from build123d import *

# Parameters (mm, degrees)
BOSS_EXTRUDE1_DEPTH = 31.75
SKETCH2_R           = 1.5
CUT_EXTRUDE1_DEPTH  = 183.851374072
FILLET1_R           = 10


with BuildPart() as part:
    # Sketch1 → Boss-Extrude1 (new body)
    with BuildSketch(Plane(origin=(0, 0, 0), x_dir=(1, 0, 0), z_dir=(0, 1, 0))):
        Polygon((0, 0), (-85, 0), (-85, 158.75), (0, 158.75), (0, 155.575), (-81.825, 155.575), (-81.825, 3.175), (0, 3.175), align=None)
    extrude(amount=BOSS_EXTRUDE1_DEPTH)

    # Sketch2 → Cut-Extrude1 (cut, through all)
    with BuildSketch(Plane.XY):
        with Locations((-7.5, 11.1125)):
            Circle(SKETCH2_R)
        with Locations((-7.5, 20.6375)):
            Circle(SKETCH2_R)
    extrude(amount=-CUT_EXTRUDE1_DEPTH, mode=Mode.SUBTRACT)

    # Fillet1
    fillet1_edges = [part.edges().sort_by_distance(p)[0] for p in [
        (-85, 15.875, 0),
        (-85, 15.875, -158.75),
        (-81.825, 15.875, -155.575),
        (-81.825, 15.875, -3.175),
    ]]
    fillet(fillet1_edges, radius=FILLET1_R)


solid = part.part
Input: part model. Units: mm. Frame: model coordinates. A direction names the side the tool comes from. Give positions to 0.01 mm unless a question says otherwise; leave off trailing zeros. Loops run counter-clockwise (first coordinate to the right, second up) from the corner with the lowest first, then second, coordinate; pieces in that order, holes last. Notation, with made-up numbers: (-2, 72) - (7, 72) arc R27 ccw to (7, 96) - close; hole circle Ø11 at (86, 21). An arc over 180 degrees is marked (long way). Use CSV: the item, a comma, the result in double quotes. Start each with the question number.
Item 1: Section D-D on z = -81. Return loops of the section in (x, y) (3 decimals).
Item 2: Line query: line 1 (Y direction, x = -7.5, z = -157.65); line 2 (Z direction, x = -37.5, y = 3.5) (3 decimals); line 3 (X direction, y = 20, z = -125) (3 decimals). Output: solid intervals per line, ascending.
Item 3: Contact query for flat-ended pins moving along their axis: P1, Ø1.5, axis at y = 3.5, z = -97, coming from the +X side (3 decimals); P2, Ø4, axis at x = -7.5, y = 11.11, coming from the -Z side. Output: stop coordinate, or through.
Item 4: Reachability of faces 1 (the flat face through (-36, 16, -3.175)), 2 (the cylindrical face through (-7.695, 22.125, -1.565)) from +Z, -Z, +X, -X, +Y, -Y: full face, straight path, thin tool, end or side. Return the list, or none.
Item 5: Mould query, pull axis Y, two halves, no side actions, for faces 3 (the flat face through (-37, 16, 0)), 4 (the cylindrical face through (-7.695, 22.125, -157.14)), 5 (the flat face through (-83, 31.75, -115)). Classes: pulls with the +Y half, pulls with the -Y half, needs draft (parallel to the pull), parting line crosses it, or undercut.
Item 6: Section B-B on x = -7.5. State how many separate pieces and enclosed holes the cut face has, then the cut area to 3 significant figures.
Item 7: Section A-A on x = -20. Return loops of the section in (y, z) (3 decimals), then the cut area to 3 significant figures.
Item 8: Section C-C on y = 6. Return loops of the section in (x, z) (3 decimals), then the cut area to 3 significant figures.
Ans:
1,outline,"(-85, 0) - (-81.825, 0) - (-81.825, 31.75) - (-85, 31.75) - close"
2,line 1,"y = 0 to 9.61, 12.61 to 19.14, 22.14 to 31.75"
2,line 2,"z = -158.75 to -155.575, -3.175 to 0"
2,line 3,"x = -85 to -81.825"
3,P1,"stops at x = -81.825"
3,P2,"stops at z = -158.75"
4,face 1,"+X, +Y, -Y"
4,face 2,"+Z, -Z"
5,face 3,"needs draft"
5,face 4,"undercut"
5,face 5,"pulls with the +Y half"
6,separate pieces,"6"
6,enclosed holes,"0"
6,area,"164 mm2"
7,outline,"(0, -158.75) - (31.75, -158.75) - (31.75, -155.575) - (0, -155.575) - close; (0, -3.175) - (31.75, -3.175) - (31.75, 0) - (0, 0) - close"
7,area,"202 mm2"
8,outline,"(-85, -148.75) arc R10 ccw to (-75, -158.75) - (0, -158.75) - (0, -155.575) - (-71.825, -155.575) arc R10 cw to (-81.825, -145.575) - (-81.825, -13.175) arc R10 cw to (-71.825, -3.175) - (0, -3.175) - (0, 0) - (-75, 0) arc R10 ccw to (-85, -10) - close"
8,area,"1,020 mm2"
